Geometry check sheet. Reference: the model listing, model coordinates, mm. A direction names the side the tool comes from. Give positions to 0.01 mm unless a question says otherwise; leave off trailing zeros. Order: outer loops, then holes, each group sorted by start corner. A loop starts at its lowest first (then second) coordinate and runs counter-clockwise, first axis right, second up. Notation, with made-up numbers: M 41,71.25 L 66,71.25 A18 cw 66,79.25 Z; hole C 18.25,27 d4. An arc over 180 degrees is marked long. Put each result on its own line as item: value. Start each with the question number.
Q1. Section check B-B on y = 2.5. Record the cut outline in (x, z), then the cut area to 3 significant figures.
Q2. Section check D-D on y = 0. Record the cut outline in (x, z).
Q3. Material ranges on L1, parallel to Z at x = 0, y = -2.5; L2, parallel to Z at x = 0.5, y = 0; L3, parallel to Y at x = -0.75, z = 4.75, recorded low to high.
Q4. Section check C-C on z = 7.25. Record the cut outline in (x, y).
Q5. Mould release check, pull along X, two halves, no side actions. Record for faces 4 (the flat face through (-1, 2, 6)), 5 (the cylindrical face through (-0.29, 1.32, 0.91)), 6 (the flat face through (0.45, 0, 9)): +X half, -X half, draft (parallel to the pull), parting line (faces both ways), or undercut.
Q6. Go/stop test with flat-tipped pins: pin 1 (2 mm diameter, centred on y = -2, z = 8.5, fed in from -X); pin 2 (1 mm diameter, centred on x = 0, y = 2, fed in from +Z); pin 3 (2 mm diameter, centred on x = 3, y = 0.5, fed in from -Z). Record where each tip stops, or that it passes through.
Q7. Section check A-A on x = 0. Record the cut outline in (y, z).
Q8. Access from +Z, -Z, +X, -X, +Y, -Y to the whole of each face (thin tool, end or side, straight path). Record for faces 1 (the flat face through (0, 0, 0)), 2 (the flat face through (-0.45, 0, 9)), 3 (the cylindrical face through (-0.38, 1.71, 4.13)).
```python
from build123d import *

# Parameters (mm, degrees)
F2_W     = 0.3
F2_H     = 0.65
F3_DEPTH = 12.5
F4_SCALE = 3


with BuildPart() as f1:
    # F0 (on Front) → F1 (revolve)
    with BuildSketch(Plane.XZ):
        Polygon((0, 3), (0, 0), (0.45, 0), (0.45, 0.6), (0.5833333333, 0.7333333333), (0.5833333333, 2), (1.25, 2), (1.25, 3), align=None)
        with BuildLine():
            Line((0, 3.2003289616), (0, 3))
            Line((0, 3), (1.25, 3))
            ThreePointArc((1.25, 3), (0.6329754523, 3.1499292043), (0, 3.2003289616))
        make_face()
    revolve(axis=Axis((0, 0, 1.5), (0, 0, -1)))

    # F2 (on Front) → F3 (cut, symmetric)
    with BuildSketch(Plane.XZ):
        with Locations((0, 2.9253289616)):
            Rectangle(F2_W, F2_H)
    extrude(amount=F3_DEPTH, both=True, mode=Mode.SUBTRACT)


with BuildPart() as f1_1:
    # F4: moved
    add(f1.part.scale(F4_SCALE))


solid = f1_1.part
```
Results found:
1. outline: M -2.8,6 L 2.8,6 L 2.8,9 A11.74 ccw 0.45,9.33 L 0.45,7.8 L -0.45,7.8 L -0.45,9.33 A11.74 ccw -2.8,9 Z
1. area: 16.7 mm^2
2. outline: M -3.75,6 L -1.75,6 L -1.75,2.2 L -1.35,1.8 L -1.35,0 L 1.35,0 L 1.35,1.8 L 1.75,2.2 L 1.75,6 L 3.75,6 L 3.75,9 A12 ccw 0.45,9.59 L 0.45,7.8 L -0.45,7.8 L -0.45,9.59 A12 ccw -3.75,9 Z
3. L1: z = 6 to 7.8
3. L2: z = 0 to 9.59
3. L3: y = -1.58 to 1.58
4. outline: C 0,0 d7.5
5. face 4: draft
5. face 5: parting line
5. face 6: undercut
6. pin 1: stops at x = -3.61
6. pin 2: stops at z = 9.46
6. pin 3: stops at z = 6
7. outline: M -3.75,6 L -1.75,6 L -1.75,2.2 L -1.35,1.8 L -1.35,0 L 1.35,0 L 1.35,1.8 L 1.75,2.2 L 1.75,6 L 3.75,6 L 3.75,7.8 L -3.75,7.8 Z
8. face 1: -Z, +X, -X, +Y, -Y
8. face 2: +Z, +Y, -Y
8. face 3: -Z
